```python
from build123d import *

# Parameters (mm, degrees)
F1_DEPTH  = 3
F4_DEPTH  = 80
F5_R      = 2
F6_DEPTH  = 80
F7_R      = 12.5
F8_DEPTH  = 3
F9_R      = 7.5
F10_DEPTH = 3.001
F12_DEPTH = 3
F15_DEPTH = 3.001
F17_DEPTH = 3.001
F18_DEPTH = 80
F13_R     = 15
F19_DEPTH = 70.1223203436
F21_DEPTH = 220
F22_R     = 12.5
F23_DEPTH = 220.001


with BuildPart() as f1:
    # F0 (on Front) → F1 (new body)
    with BuildSketch(Plane.XZ):
        Polygon((-93.6853438616, -3.4913793206), (286.3146561384, -3.4913793206), (286.3146561384, 116.5086206794), (228.8437245958, 116.5086206794), (-93.6853438616, 76.5086206794), align=None)
    extrude(amount=F1_DEPTH)

    # F2 (on face) → F4 (join)
    with BuildSketch(Plane(origin=(0, 0, -3.4913793206), x_dir=(1, 0, 0), z_dir=(0, 0, -1))):
        Polygon((-185.6092254158, 94.9238815543), (-93.6853438616, 3), (-89.4427031745, 3), (-183.4879050723, 97.0452018978), align=None)
    extrude(amount=-F4_DEPTH)

    # F5
    f5_edges = [f1.edges().sort_by_distance(p)[0] for p in [
        (-93.685344, 0, 36.508621),
    ]]
    fillet(f5_edges, radius=F5_R)

    # F7 (on face) → F8 (cut)
    with BuildSketch(Plane.XZ.offset(3)):
        with Locations((124.0946352482, 54.7083429992)):
            Circle(F7_R)
    extrude(amount=-F8_DEPTH, mode=Mode.SUBTRACT)

    # F9 (on face) → F10 (cut, through all)
    with BuildSketch(Plane.XZ.offset(3)):
        with Locations((-32.7149666846, 42.6947064698)):
            Circle(F9_R)
    extrude(amount=-F10_DEPTH, mode=Mode.SUBTRACT)

    # F11 (on face) → F12 (cut)
    with BuildSketch(Plane.XZ.offset(3)):
        with BuildLine():
            ThreePointArc((-25.2149666846, 42.6947064698), (-27.0880889677, 37.736052705), (-31.7718325937, 35.2542429031))
            Line((-31.7718325937, 35.2542429031), (124.6507872105, 42.2207213283))
            ThreePointArc((124.6507872105, 42.2207213283), (111.6310963493, 53.754299962), (122.7436713431, 67.1351244219))
            Line((122.7436713431, 67.1351244219), (-33.2737348604, 50.173862714))
            ThreePointArc((-33.2737348604, 50.173862714), (-27.6130435824, 48.192013143), (-25.2149666846, 42.6947064698))
        make_face()
    extrude(amount=-F12_DEPTH, mode=Mode.SUBTRACT)

    # F14 (on face) → F15 (cut, through all)
    with BuildSketch(Plane.XZ.offset(3)):
        with BuildLine():
            ThreePointArc((239.3146561384, 106.0872673988), (238.435976482, 108.2085877424), (236.3146561384, 109.0872673988))
            ThreePointArc((236.3146561384, 109.0872673988), (234.1933357949, 103.9659470553), (239.3146561384, 106.0872673988))
        make_face()
    extrude(amount=-F15_DEPTH, mode=Mode.SUBTRACT)

    # F16 (on face) → F17 (cut, through all)
    with BuildSketch(Plane.XZ.offset(3)):
        with BuildLine():
            ThreePointArc((239.3146561384, 6.0872673988), (238.435976482, 8.2085877424), (236.3146561384, 9.0872673988))
            ThreePointArc((236.3146561384, 9.0872673988), (234.1933357949, 3.9659470553), (239.3146561384, 6.0872673988))
        make_face()
    extrude(amount=-F17_DEPTH, mode=Mode.SUBTRACT)



with BuildPart() as f6:
    # F3 (on face) → F6 (new body)
    with BuildSketch(Plane(origin=(0, 0, -3.4913793206), x_dir=(1, 0, 0), z_dir=(0, 0, -1))):
        Polygon((-183.4879050723, 97.0452018978), (-185.6092254158, 94.9238815543), (-93.6853438616, 3), (-89.4427031745, 3), align=None)
    extrude(amount=-F6_DEPTH)


with BuildPart() as f1_1:
    add(f1.part)

    add(f6.part)  # F18 merges F6
    # F2 (on face) → F18 (join)
    with BuildSketch(Plane(origin=(0, 0, -3.4913793206), x_dir=(1, 0, 0), z_dir=(0, 0, -1))):
        Polygon((-185.6092254158, 94.9238815543), (-93.6853438616, 3), (-89.4427031745, 3), (-183.4879050723, 97.0452018978), align=None)
    extrude(amount=-F18_DEPTH)

    # F13 (on face) → F19 (cut, through all)
    with BuildSketch(Plane(origin=(-43.2213515872, 43.2213515872, 0), x_dir=(0.7071067812, 0.7071067812, 0), z_dir=(0.7071067812, -0.7071067812, 0))):
        with Locations((-138.838544488, 39.6711453795)):
            Circle(F13_R)
    extrude(amount=-F19_DEPTH, mode=Mode.SUBTRACT)

    # F20 (on face) → F21 (join)
    with BuildSketch(Plane.XY.offset(76.5086206794)):
        with BuildLine():
            Line((-184.5485652441, -95.984541726), (-184.0766972591, -96.456409711))
            ThreePointArc((-184.0766972591, -96.456409711), (-184.3103818476, -96.2182263145), (-184.5485652441, -95.984541726))
        make_face()
        with BuildLine():
            ThreePointArc((-184.5485652441, -95.984541726), (-212.7880613937, -115.4433890159), (-179.1847505183, -108.5925949853))
            ThreePointArc((-179.1847505183, -108.5925949853), (-180.4537472832, -102.0500775813), (-184.0766972591, -96.456409711))
            Line((-184.0766972591, -96.456409711), (-184.5485652441, -95.984541726))
        make_face()
    extrude(amount=-F21_DEPTH)

    # F22 (on face) → F23 (cut, through all)
    with BuildSketch(Plane.XY.offset(76.5086206794)):
        with Locations((-196.6847505183, -108.5925949853)):
            Circle(F22_R)
    extrude(amount=-F23_DEPTH, mode=Mode.SUBTRACT)


with BuildPart() as f24_1:
    # F24: instance of F1
    add(f1_1.part.mirror(Plane.YZ))


solid = f1_1.part
```
Could you check a few things on this model? Use its own coordinates, in mm. A direction names the side the tool comes from. Round coordinates to 2 decimals unless told otherwise and drop trailing zeros. Loops run counter-clockwise (first coordinate to the right, second up) from the corner with the lowest first, then second, coordinate; pieces in that order, holes last. Notation, with made-up numbers: (-1, 21) -> (41, 21) arc R21 ccw to (41, 27) -> close; hole circle Ø1 at (-5, 4). An arc over 180 degrees is marked (long way). Put each result on its own line as item: value.
Q1. I want a section at A-A on x = -13. Write out the boundary of the cut face in (y, z).
Checks:
outline: (-3, -3.49) -> (0, -3.49) -> (0, 36.09) -> (-3, 36.09) -> close; (-3, 52.38) -> (0, 52.38) -> (0, 86.52) -> (-3, 86.52) -> close
Q2. I want a section at D-D on z = 88. Write out the boundary of the cut face in (x, y).
Checks:
outline: (-1.03, -3) -> (286.31, -3) -> (286.31, 0) -> (-1.03, 0) -> close
Q3. I want a section at B-B on z = 15. Write out the boundary of the cut face in (x, y), and give its area (3 significant figures).
Checks:
outline: (-185.61, -94.92) -> (-184.55, -95.98) arc R17.5 ccw (long way) to (-184.08, -96.46) -> (-183.49, -97.05) -> (-89.44, -3) -> (286.31, -3) -> (286.31, 0) -> (-91.69, 0) arc R2 ccw to (-93.69, -2) -> (-93.69, -3) -> close; hole circle Ø25 at (-196.68, -108.59)
area: 2,000 mm2
Q4. Please list where these lines run through material, in increasing order: line 1 (Y direction, x = 200, z = 98); line 2 (Y direction, x = -192, z = -129); line 3 (X direction, y = -99, z = 67.5). Write a range as from..to.
Checks:
line 1: -3..0
line 2: -125.45..-120.18, -97..-91.73
line 3: -211.32..-204.7, -188.67..-182.05
Q5. Thinking about a two-plate mould opening in X: for faces 1 (the flat face through (136, -3, 44)), 2 (the cylindrical face through (136.576, -1.521, 55.383)), 3 (the flat face through (-125.358, -38.915, 35.949)), 4 (the cylindrical face through (-185.14, -113.38, -31.95)), which applies, pulls with the +X half, pulls with the -X half, needs draft (parallel to the pull), parting line crosses it, or undercut?
Checks:
face 1: needs draft
face 2: undercut
face 3: pulls with the +X half
face 4: undercut
Q6. I want a section at C-C on y = -30.5. Write out the boundary of the cut face in (x, z), and give its area (3 significant figures).
Checks:
outline: (-121.19, -3.49) -> (-116.94, -3.49) -> (-116.94, 76.51) -> (-121.19, 76.51) -> close
area: 339 mm2
Q7. Which directions (+Z, -Z, +X, -X, +Y, -Y) give clear straight access to the entire face, cutting with the end or side of a thin tool? Please do faces 5 (the flat face through (45.827, -1.521, 58.773)), 6 (the flat face through (69.84, -1.48, 96.79)).
Checks:
face 5: +Y, -Y
face 6: +Z, -X, +Y, -Y
Q8. For pin 1 Ø1.1 at (y, z) = (-2.5, 19) entering from -X, with a flat end and sliding along its axis, tell me the tip position at first contact or that it passes through.
Checks:
pin 1: x = -93.74
